from build123d import *

# Parameters (mm, degrees)
F0_W     = 52.7686178684
F0_H     = 46.8310452998
F1_DEPTH = 45.0226236135
F2_W     = 61.3688528538
F2_H     = 15.6810022891
F3_DEPTH = 27.3912083358
F4_DEPTH = 109.2513594776
F5_DEPTH = 59.5592800528


# Not quite as in the source:
# - a feature names something its author has since deleted; it is built from what else it names


with BuildPart() as f1:
    # F0 (on Front) → F1 (new body)
    with BuildSketch(Plane.XZ):
        with Locations((26.3843089342, 23.4155226499)):
            Rectangle(F0_W, F0_H)
    extrude(amount=F1_DEPTH)

    # F2 (on Right) → F3 (join)
    with BuildSketch(Plane.YZ):
        with Locations((-47.6985424757, 54.6393077821)):
            Rectangle(F2_W, F2_H)
    extrude(amount=F3_DEPTH)

    # F4 (add): a face of the model
    f4_faces = [f1.faces().sort_by_distance(p)[0] for p in [
        (52.7686178684, -22.5113118067, 23.4155226499),
    ]]
    extrude(f4_faces, amount=F4_DEPTH)

    # F5 (add): a face of the model
    f5_faces = [f1.faces().sort_by_distance(p)[0] for p in [
        (81.009988673, 0, 23.4155226499),
    ]]
    extrude(f5_faces, amount=F5_DEPTH)


solid = f1.part
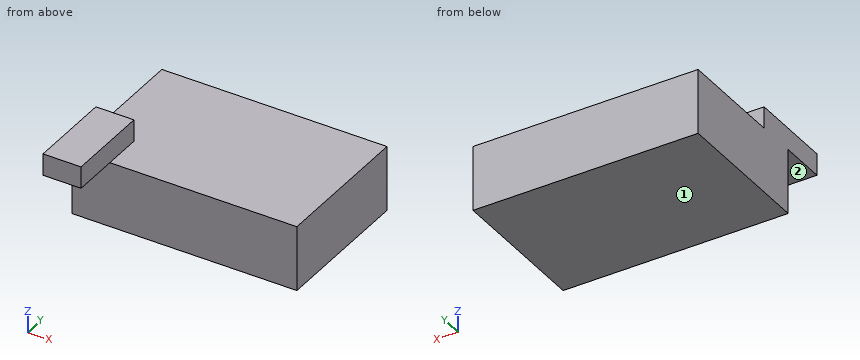
The listing builds one solid part. Answer for the finished solid, in the listing's coordinates (mm). Face numbers are marked on the shaded views. A direction names the side the tool comes from. Round coordinates to 2 decimals unless told otherwise and drop trailing zeros. Write each loop counter-clockwise with the first axis right and the second up, starting at its lowest first coordinate (ties: lowest second). Pieces come first, ordered by that corner, then holes. Notation, with made-up numbers: M -31,-12 L 0,-12 A20 cw 0,-7 Z; hole C -22,55 d8. An arc over 180 degrees is marked long. Write each question's results on one line, items separated by ' | '. Start each with the question number.
(1) The part is cut by section C-C, the plane x = 113. Write down the section's boundary in (y, z), and give its area (3 significant figures).
(2) Each of these flat-tipped pins is pushed along its axis until it touches: P1, Ø1.5, axis at x = 47.5, z = 38.5, coming from the -Y side; P2, Ø4.5, axis at y = -59.5, z = 53, coming from the +X side; P3, Ø12, axis at x = 86, y = -53.5, coming from the -Z side; P4, Ø1.5, axis at x = 106, y = -42.5, coming from the -Z side. Where does it stop, or does it pass through?
(3) For the marked faces 1 and 2, determine the directions among +Z, -Z, +X, -X, +Y, -Y from which every point of the face is accessible in a straight line to the end or side of a thin tool.
(4) Find the intervals of material crossed by line 1 (Y direction, x = 66, z = 29.5); line 2 (Z direction, x = 140.5, y = 52); line 3 (Y direction, x = 11.5, z = 47), in increasing order.
(5) The part is cut by section B-B, the plane z = 18.5. Write down the section's boundary in (x, y).
(6) The part is cut by section A-A, the plane y = -25.5. Write down the section's boundary in (x, z).
Worked answers:
1) outline: M -45.02,0 L 59.56,0 L 59.56,46.83 L -45.02,46.83 Z | area: 4,900 mm²
2) P1: stops at y = -45.02 | P2: stops at x = 27.39 | P3: passes through | P4: stops at z = 0
3) face 1: -Z, +X, -X, +Y, -Y | face 2: -Z, +X, -X, -Y
4) line 1: y = -45.02 to 59.56 | line 2: z = 0 to 46.83 | line 3: y = -78.38 to -17.01
5) outline: M 0,-45.02 L 162.02,-45.02 L 162.02,59.56 L 0,59.56 Z
6) outline: M 0,0 L 162.02,0 L 162.02,46.83 L 27.39,46.83 L 27.39,62.48 L 0,62.48 Z
